For this review, take the finished solid that the model builds, in its own axes (mm). Give positions to 0.01 mm unless a question says otherwise; leave off trailing zeros. Write each loop counter-clockwise with the first axis right and the second up, starting at its lowest first coordinate (ties: lowest second). Pieces come first, ordered by that corner, then holes. Notation, with made-up numbers: (66.5, 44.5) -> (115.5, 44.5) arc R18 ccw to (115.5, 77.5) -> close; hole circle Ø6 at (87, -4.75). An arc over 180 degrees is marked (long way). Write item = value, one per line.
```python
from build123d import *

# Parameters (mm, degrees)
F0_W     = 60
F0_H     = 46.85
F0_R     = 2.75
F0_R_2   = 1.6
F1_DEPTH = 3
F2_SIZE  = 2


with BuildPart() as f1:
    # F0 (on Front) → F1 (new body)
    with BuildSketch(Plane.XZ):
        with Locations((30, 23.425)):
            Rectangle(F0_W, F0_H)
        with Locations((15, 12.7)):
            Circle(F0_R, mode=Mode.SUBTRACT)
        with Locations((45, 12.7)):
            Circle(F0_R, mode=Mode.SUBTRACT)
        with Locations((14.5, 42.4)):
            Circle(F0_R_2, mode=Mode.SUBTRACT)
        with Locations((45.5, 42.4)):
            Circle(F0_R_2, mode=Mode.SUBTRACT)
    extrude(amount=-F1_DEPTH)

    # F2
    f2_edges = [f1.edges().sort_by_distance(p)[0] for p in [
        (0, 1.5, 46.85),
        (0, 1.5, 0),
        (60, 1.5, 0),
        (60, 1.5, 46.85),
    ]]
    chamfer(f2_edges, length=F2_SIZE)


solid = f1.part
```
(1) Take a section at A-A (z = 42.4). Write out the cut boundary in (x, y).
Answers below:
outline = (0, 0) -> (12.9, 0) -> (12.9, 3) -> (0, 3) -> close; (16.1, 0) -> (43.9, 0) -> (43.9, 3) -> (16.1, 3) -> close; (47.1, 0) -> (60, 0) -> (60, 3) -> (47.1, 3) -> close
(2) To check wall thickness, follow probe 1 along Z at (x, y) = (14.5, 1.4); probe 2 along Z at (x, y) = (45, 0.95); probe 3 along X at (y, z) = (2.9, 14.5). State the ranges of each line that lie inside material, in increasing order.
Answers below:
probe_1 = 0 to 10, 15.4 to 40.8, 44 to 46.85
probe_2 = 0 to 9.95, 15.45 to 40.88, 43.92 to 46.85
probe_3 = 0 to 12.92, 17.08 to 42.92, 47.08 to 60
(3) The part is to be moulded in two halves that separate along X. For faces 1 (the face through (42.253, 1.479, 12.821)), 2 (the face through (30, 3, 24)), 3 (the face through (1.01, 1.48, 45.86)), say which applies: released by +X, released by -X, zero draft, split by the parting line, or undercut.
Answers below:
face_1 = undercut
face_2 = zero draft
face_3 = released by -X
(4) For pin 1 (1 mm diameter, centred on x = 53, z = 18, fed in from -Y), flat-tipped, find the tip position at first contact; note if it passes through.
Answers below:
pin_1 = 0
(5) Take a section at B-B (x = 45.5). Write out the cut boundary in (y, z).
Answers below:
outline = (0, 0) -> (3, 0) -> (3, 10) -> (0, 10) -> close; (0, 15.4) -> (3, 15.4) -> (3, 40.8) -> (0, 40.8) -> close; (0, 44) -> (3, 44) -> (3, 46.85) -> (0, 46.85) -> close
(6) Take a section at C-C (y = 1). Write out the cut boundary in (x, z), plus the area to 3 significant figures.
Answers below:
outline = (0, 2) -> (2, 0) -> (58, 0) -> (60, 2) -> (60, 44.85) -> (58, 46.85) -> (2, 46.85) -> (0, 44.85) -> close; hole circle Ø5.5 at (15, 12.7); hole circle Ø3.2 at (14.5, 42.4); hole circle Ø5.5 at (45, 12.7); hole circle Ø3.2 at (45.5, 42.4)
area = 2,740 mm^2
